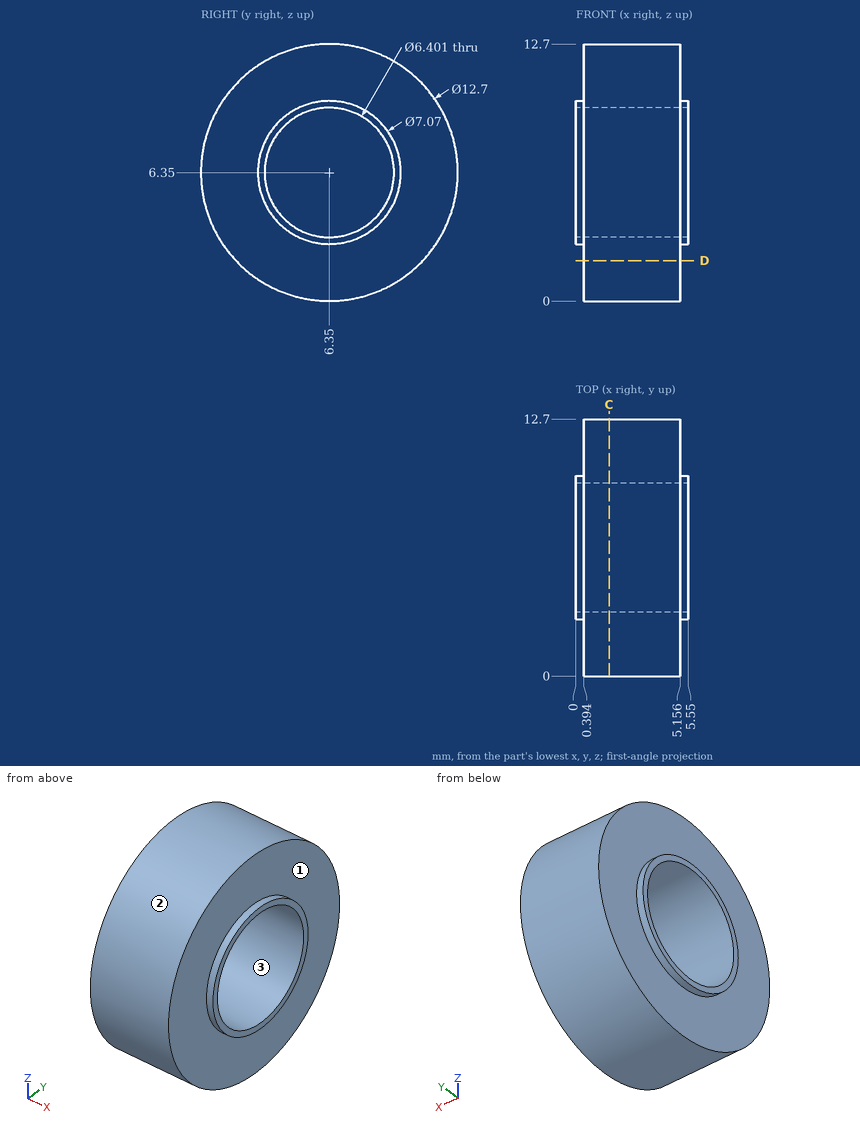
Geometry: see drawing. Coordinates: mm, zero at the bounding-box minimum. Give positions to 0.01 mm unless a question says otherwise; leave off trailing zeros. Order: outer loops, then holes, each group sorted by start corner. A loop starts at its lowest first (then second) coordinate and runs counter-clockwise, first axis right, second up.
1. Draft query along Z for the marked faces 1, 2 and 3. Return one class per face: released by +Z, released by -Z, zero draft, split by the parting line, or undercut.
Computed:
face 1: zero draft
face 2: split by the parting line
face 3: undercut
2. Cut plane D-D (z = 2). Return loops of the section in (x, y).
Computed:
outline: (0.39, 1.72) - (5.16, 1.72) - (5.16, 10.98) - (0.39, 10.98) - close
3. Pin query (flat end, axial travel): pin 1 Ø1 at (y, z) = (4.5, 5) entering from -X; pin 2 Ø2 at (x, z) = (4, 3) entering from +Y; pin 3 Ø3 at (x, z) = (2, 4) entering from +Y. Return the tip coordinate at first contact, or that it passes through.
Computed:
pin 1: passes through
pin 2: stops at y = 12.25
pin 3: stops at y = 12.64
4. Cut plane C-C (x = 1.65). Return loops of the section in (y, z).
Computed:
outline: circle Ø12.7 at (6.35, 6.35); hole circle Ø6.4 at (6.35, 6.35)
5. Line query: probe 1 along Z at (x, y) = (2.7, 6.35); probe 2 along X at (y, z) = (1.25, 6); probe 3 along Z at (x, y) = (4.85, 5.5) (1 decimal). Output: solid intervals per line, ascending.
Computed:
probe 1: z = 0 to 3.15, 9.55 to 12.7
probe 2: x = 0.39 to 5.16
probe 3: z = 0.1 to 3.3, 9.4 to 12.6
